```python
from build123d import *

# Parameters (mm, degrees)
SKETCH1_R           = 7.9375
BOSS_EXTRUDE1_DEPTH = 101.6
CUT_EXTRUDE1_DEPTH  = 153.4
SKETCH3_R           = 5.1562
CUT_EXTRUDE2_DEPTH  = 150.32089472
SKETCH4_R           = 5.903408011
CUT_EXTRUDE3_DEPTH  = 131.136274728
FILLET1_R           = 10.16


with BuildPart() as part:
    # Sketch1 → Boss-Extrude1 (new body)
    with BuildSketch(Plane(origin=(0, 0, 0), x_dir=(1, 0, 0), z_dir=(0, 1, 0))):
        with BuildLine():
            Line((0, 0), (-76.2, 0))
            ThreePointArc((-76.2, 0), (-101.6, -25.4), (-76.2, -50.8))
            Line((-76.2, -50.8), (-38.1, -50.8))
            Line((-38.1, -50.8), (-38.1, -10.16))
            Line((-38.1, -10.16), (0, -10.16))
            Line((0, -10.16), (0, 0))
        make_face()
        with Locations(Location((-76.2, -25.4, 0), (0, 0, 270))):
            Circle(SKETCH1_R, mode=Mode.SUBTRACT)
    extrude(amount=-BOSS_EXTRUDE1_DEPTH)

    # Sketch2 → Cut-Extrude1 (cut, through all)
    with BuildSketch(Plane.XY.offset(50.8)):
        with BuildLine():
            Line((-53.34, -17.78), (-111.029892198, -17.78))
            Line((-111.029892198, -17.78), (-111.029892198, -83.82))
            Line((-111.029892198, -83.82), (-53.34, -83.82))
            ThreePointArc((-53.34, -83.82), (-49.747897552, -82.332102448), (-48.26, -78.74))
            Line((-48.26, -78.74), (-48.26, -22.86))
            ThreePointArc((-48.26, -22.86), (-49.747897552, -19.267897552), (-53.34, -17.78))
        make_face()
    extrude(amount=-CUT_EXTRUDE1_DEPTH, mode=Mode.SUBTRACT)

    # Sketch3 → Cut-Extrude2 (cut, through all)
    with BuildSketch(Plane.XY.offset(10.16)):
        with Locations((-20.32, -15.24)):
            Circle(SKETCH3_R)
        with Locations((-20.32, -86.36)):
            Circle(SKETCH3_R)
    extrude(amount=-CUT_EXTRUDE2_DEPTH, mode=Mode.SUBTRACT)

    # Sketch4 → Cut-Extrude3 (cut, through all)
    with BuildSketch(Plane(origin=(-38.1, 0, 0), x_dir=(0, 0, -1), z_dir=(1, 0, 0))):
        with Locations((-27.94, -50.8)):
            Circle(SKETCH4_R)
    extrude(amount=-CUT_EXTRUDE3_DEPTH, mode=Mode.SUBTRACT)

    # Fillet1
    fillet1_edges = [part.edges().sort_by_distance(p)[0] for p in [
        (0, -101.6, 5.08),
        (0, 0, 5.08),
    ]]
    fillet(fillet1_edges, radius=FILLET1_R)


solid = part.part
```
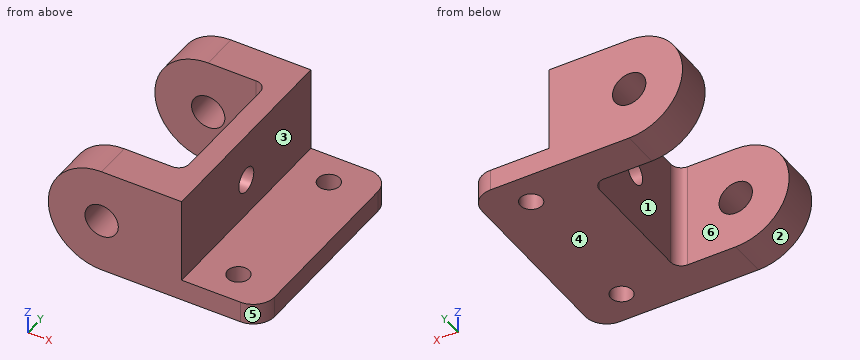
Geometry: final body of the model. Coordinates: model frame, mm. Face numbers are marked on the shaded views. A direction names the side the tool comes from. Round coordinates to 2 decimals unless told otherwise and drop trailing zeros. Write each loop counter-clockwise with the first axis right and the second up, starting at its lowest first coordinate (ties: lowest second). Pieces come first, ordered by that corner, then holes. Notation, with made-up numbers: M -28.5,-19 L -24.5,-19 A30 ccw -24.5,10 Z; hole C -10,-38.5 d8. An arc over 180 degrees is marked long. Answer in a Markdown table with one row per item. Add a question column.
(1) Cut plane C-C, the plane x = -20.32. Return the cut outline in (y, z).
(2) Ray query, L1, parallel to Y at x = -20.32, z = 5.25; L2, parallel to Y at x = -59, z = 6; L3, parallel to Z at x = -15.5, y = -24.5. Return the intervals inside material, ascending.
(3) Cut plane D-D, the plane z = 27. Return the cut outline in (x, y).
(4) Cut plane B-B, the plane y = -50.8. Return the cut outline in (x, z), then the cut area to 3 significant figures.
(5) Contact query for flat-ended pins moving along their axis: pin 1 (19 mm diameter, centred on x = -14, y = -66, fed in from +Z); pin 2 (6 mm diameter, centred on y = -45.5, z = 21, fed in from -X); pin 3 (8 mm diameter, centred on x = -35.5, z = 18, fed in from -Y). Output: stop coordinate, or through.
(6) Cut plane A-A, the plane y = -15.24. Return the cut outline in (x, z) (1 decimal), then the cut area to 3 significant figures.
(7) Draft query along Y for the marked faces 4, 5 and 6. Return one class per face: pulls with the +Y half, pulls with the -Y half, needs draft (parallel to the pull), parting line crosses it, or undercut.
(8) Reachability of the marked faces 1, 2 and 3 from +Z, -Z, +X, -X, +Y, -Y: full face, straight path, thin tool, end or side. Return the list, or none.
Established:
| question | item | result |
|---|---|---|
| 1 | outline | M -101.6,0 L -91.52,0 L -91.52,10.16 L -101.6,10.16 Z; M -81.2,0 L -20.4,0 L -20.4,10.16 L -81.2,10.16 Z; M -10.08,0 L 0,0 L 0,10.16 L -10.08,10.16 Z |
| 2 | L1 | -101.6 to -91.52, -81.2 to -20.4, -10.08 to 0 |
| 2 | L2 | -101.6 to -83.82, -17.78 to 0 |
| 2 | L3 | 0 to 10.16 |
| 3 | outline | M -101.55,-101.6 L -83.97,-101.6 L -83.97,-83.82 L -101.55,-83.82 Z; M -101.55,-17.78 L -83.97,-17.78 L -83.97,0 L -101.55,0 Z; M -68.43,-101.6 L -38.1,-101.6 L -38.1,-56.63 L -48.26,-56.63 L -48.26,-78.74 A5.08 cw -53.34,-83.82 L -68.43,-83.82 Z; M -68.43,-17.78 L -53.34,-17.78 A5.08 cw -48.26,-22.86 L -48.26,-44.97 L -38.1,-44.97 L -38.1,0 L -68.43,0 Z |
| 4 | outline | M -48.26,0 L 0,0 L 0,10.16 L -38.1,10.16 L -38.1,22.04 L -48.26,22.04 Z; M -48.26,33.84 L -38.1,33.84 L -38.1,50.8 L -48.26,50.8 Z |
| 4 | area | 783 mm² |
| 5 | pin 1 | z = 10.16 |
| 5 | pin 2 | x = -48.26 |
| 5 | pin 3 | y = -101.6 |
| 6 | outline | M -76.2,0 L -25.5,0 L -25.5,10.2 L -38.1,10.2 L -38.1,50.8 L -76.2,50.8 A25.4 ccw Z; M -15.2,0 L 0,0 L 0,10.2 L -15.2,10.2 Z; hole C -76.2,25.4 d15.9 |
| 6 | area | 3,030 mm² |
| 7 | face 4 | needs draft |
| 7 | face 5 | pulls with the -Y half |
| 7 | face 6 | undercut |
| 8 | face 1 | +Z, -Z, -X |
| 8 | face 2 | -X, +Y, -Y |
| 8 | face 3 | +Z, +X, +Y, -Y |
